Study the drawing (mm; zero at the part's minimum x, y, z) and answer. A direction names the side the tool comes from. Give positions to 0.01 mm unless a question says otherwise; leave off trailing zeros. Loops run counter-clockwise (first coordinate to the right, second up) from the corner with the lowest first, then second, coordinate; pieces in that order, holes last. Notation, with made-up numbers: (13, -21.75) -> (61, -21.75) arc R23 ccw to (61, 17.25) -> close; hole circle Ø10 at (77, 24). An arc over 180 degrees is marked (long way). One line per question, with ' | ' between items. Start each with the question number.
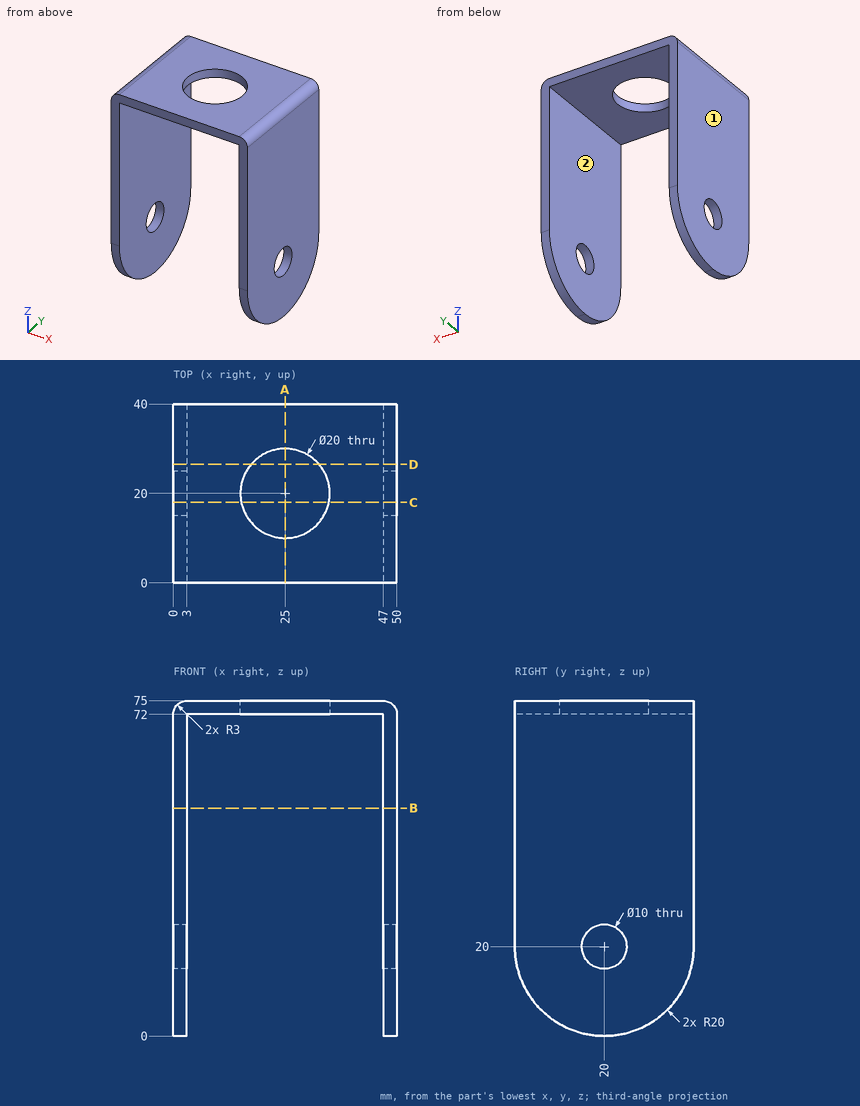
1. The part is cut by section B-B (z = 51). Write down the section's boundary in (x, y), plus the area to 3 significant figures.
2. The part is cut by section A-A (x = 25). Write down the section's boundary in (y, z), plus the area to 3 significant figures.
3. The part is cut by section D-D (y = 26.5). Write down the section's boundary in (x, z).
4. Each of these flat-tipped pins is pushed along its axis until it touches: pin 1 Ø12 at (x, z) = (37, 61) entering from +Y; pin 2 Ø20 at (y, z) = (28.5, 28) entering from -X. Where does it stop, or does it pass through?
5. For the marked faces 1 and 2, determine the directions among +Z, -Z, +X, -X, +Y, -Y from which every point of the face is accessible in a straight line to the end or side of a thin tool.
6. Straight lines are drawn through the part: L1, parallel to X at y = 13, z = 44; L2, parallel to Y at x = 1.8, z = 20; L3, parallel to Y at x = 25, z = 73. For each, find the intervals that lie inside material, in ascending order.
7. The part is cut by section C-C (y = 18). Write down the section's boundary in (x, z).
Check sheet entries:
1) outline: (0, 0) -> (3, 0) -> (3, 40) -> (0, 40) -> close; (47, 0) -> (50, 0) -> (50, 40) -> (47, 40) -> close | area: 240 mm^2
2) outline: (0, 72) -> (10, 72) -> (10, 75) -> (0, 75) -> close; (30, 72) -> (40, 72) -> (40, 75) -> (30, 75) -> close | area: 60.0 mm^2
3) outline: (0, 1.09) -> (3, 1.09) -> (3, 72) -> (17.4, 72) -> (17.4, 75) -> (3, 75) arc R3 ccw to (0, 72) -> close; (32.6, 72) -> (47, 72) -> (47, 1.09) -> (50, 1.09) -> (50, 72) arc R3 ccw to (47, 75) -> (32.6, 75) -> close
4) pin 1: passes through | pin 2: stops at x = 0
5) face 1: +Z, -Z, -X, +Y, -Y | face 2: -Z, +Y, -Y
6) L1: x = 0 to 3, 47 to 50 | L2: y = 0 to 15, 25 to 40 | L3: y = 0 to 10, 30 to 40
7) outline: (0, 0.1) -> (3, 0.1) -> (3, 15.42) -> (0, 15.42) -> close; (0, 24.58) -> (3, 24.58) -> (3, 72) -> (15.2, 72) -> (15.2, 75) -> (3, 75) arc R3 ccw to (0, 72) -> close; (34.8, 72) -> (47, 72) -> (47, 24.58) -> (50, 24.58) -> (50, 72) arc R3 ccw to (47, 75) -> (34.8, 75) -> close; (47, 0.1) -> (50, 0.1) -> (50, 15.42) -> (47, 15.42) -> close
